Read the model definition and answer for the solid it produces. Units are mm, in the model's axes. Face numbers are marked on the shaded views. A direction names the side the tool comes from. Give positions to 0.01 mm unless a question says otherwise; leave off trailing zeros. Order: outer loops, then holes, each group sorted by start corner. A loop starts at its lowest first (then second) coordinate and runs counter-clockwise, first axis right, second up. Notation, with made-up numbers: (55, 56) -> (100, 56) arc R24 ccw to (100, 95) -> close; hole circle Ø2 at (-12.75, -24.75). An arc over 180 degrees is marked (long way). One line per item, written item: value. Start each with the question number.
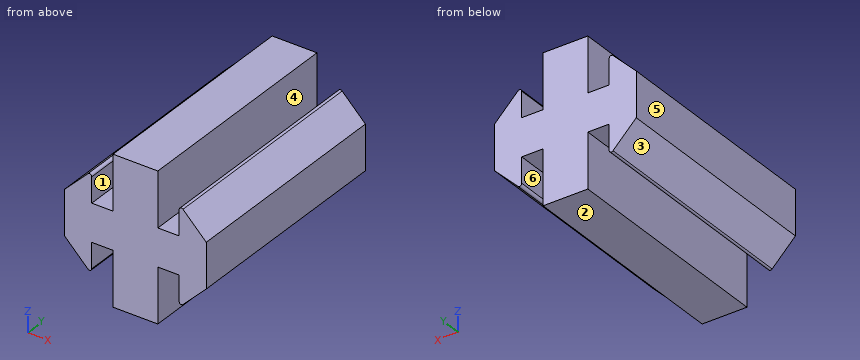
Autodesk Inventor part; units mm, degrees
ref_plane "YZ Plane" through (0, 0, 0) normal (1, 0, 0) x (0, 1, 0)
ref_plane "XZ Plane" through (0, 0, 0) normal (0, 1, 0) x (-1, 0, 0)
ref_plane "XY Plane" through (0, 0, 0) normal (0, 0, 1) x (1, 0, 0)
sketch "Sketch1" plane through (0, 0, 0) normal (0, 1, 0) x (-1, 0, 0)
  line L0 (0, 0) -> (5.08, 0)
  line L1 (5.08, 0) -> (5.08, -16.637)
  line L2 (5.08, -16.637) -> (0, -16.637)
  line L3 (0, -16.637) -> (0, 0)
  line L4 (0, -6.1892) -> (7.493, -6.1892)
  line L5 (7.493, -6.1892) -> (7.493, -10.4478)
  line L6 (7.493, -10.4478) -> (0, -10.4478)
  line L7 (10.5664, -5.7785) -> (10.5664, -10.8585)
  line L8 (7.493, -13.9319) -> (7.493, -2.7051)
  line L9 (7.493, -13.9319) -> (10.5664, -10.8585)
  line L10 (7.493, -2.7051) -> (10.5664, -5.7785)
  line L11 (0, -6.1892) -> (-2.413, -6.1892)
  line L12 (-2.413, -10.4478) -> (0, -10.4478)
  line L13 (-5.4864, -5.7785) -> (-5.4864, -10.8585)
  line L14 (-2.413, -13.9319) -> (-2.413, -2.7051)
  line L15 (-2.413, -13.9319) -> (-5.4864, -10.8585)
  line L16 (-2.413, -2.7051) -> (-5.4864, -5.7785)
  point P0 (-4.9276, -6.1892)
  dimension "d0" = 5.08
  dimension "d1" = 16.637
  dimension "d2" = 2.413
  dimension "d9" = 3.0734
  dimension "d12" = 0
  dimension "d16" = 11.2268
  dimension "d20" = 135
  dimension "d21" = 135
  dimension "d24" = 6.1893
  dimension "d25" = 16.637
  dimension "d26" = 3.4842
  dimension "d33" = 3.4842
  dimension "d34" = 3.0734
  dimension "d35" = 2.413
  dimension "d36" = 6.1893
  dimension "d37" = 5.08
  dimension "d38" = 5.08
  dimension "d39" = 135
  dimension "d40" = 135
extrude "Extrusion2" add sketch "Sketch1" along normal blind 25.4
fillet "Fillet1" radius 0.254 4 edges at (2.413, 12.7, -13.9319) (-7.493, 12.7, -13.9319) (2.413, 12.7, -2.7051) (-7.493, 12.7, -2.7051)
equation "\"d16\" = d15"
equation "\"d21\" = d20"
equation "\"d24\" = -0.5 * d4 + 0.5 * d25"
properties part number "20X20 lift conecter" material "PC/ABS Plastic"
Item 1: For a pull along X with two mould halves and no side action, classify the marked faces 1, 2 and 3 as +X half, -X half, draft (parallel to the pull), parting line (faces both ways), or undercut.
Item 2: Find section D-D on z = -14. Write down the section's boundary in (x, y), then the cut area to 3 significant figures.
Item 3: Find section C-C on x = -5.5. Write down the section's boundary in (y, z), then the cut area to 3 significant figures.
Item 4: Find the intervals of material crossed by line 1 (X direction, y = 10, z = -6); line 2 (X direction, y = 23.5, z = -5); line 3 (X direction, y = 20.75, z = -3), in increasing order. Write a range as from..to.
Item 5: Find section A-A on z = -5.5. Write down the section's boundary in (x, y), then the cut area to 3 significant figures.
Item 6: Find section B-B on y = 4.5. Write down the section's boundary in (x, z).
Item 7: A tool of negligible diameter and unlimited length cuts with its end or side. For the marked faces 4, 5 and 6, from which of +Z, -Z, +X, -X, +Y, -Y can it reach the whole face along a straight path? Write none if from no direction.
Item 8: Flat-ended cylindrical pins translate along their axes: pin 1 (1.5 mm diameter, centred on x = -4.5, y = 15, fed in from +Z); pin 2 (0.7 mm diameter, centred on x = 1, y = 11.5, fed in from -Z); pin 3 (1 mm diameter, centred on x = 2.5, y = 20, fed in from +Z); pin 4 (0.9 mm diameter, centred on y = 10.5, z = -4.5, fed in from +X). Find the tip coordinate at first contact, or state that the pin passes through.
Checks:
1. face 1: undercut
1. face 2: draft
1. face 3: -X half
2. outline: (-5.08, 0) -> (0, 0) -> (0, 25.4) -> (-5.08, 25.4) -> close
2. area: 129 mm2
3. outline: (0, -10.45) -> (25.4, -10.45) -> (25.4, -6.19) -> (0, -6.19) -> close
3. area: 108 mm2
4. line 1: -10.57..-7.49, -5.08..0, 2.41..5.49
4. line 2: -9.79..-7.49, -5.08..0, 2.41..4.71
4. line 3: -5.08..0
5. outline: (-10.29, 0) -> (-7.49, 0) -> (-7.49, 25.4) -> (-10.29, 25.4) -> close; (-5.08, 0) -> (0, 0) -> (0, 25.4) -> (-5.08, 25.4) -> close; (2.41, 0) -> (5.21, 0) -> (5.21, 25.4) -> (2.41, 25.4) -> close
5. area: 271 mm2
6. outline: (-10.57, -10.86) -> (-7.93, -13.5) arc R0.25 ccw to (-7.49, -13.32) -> (-7.49, -10.45) -> (-5.08, -10.45) -> (-5.08, -16.64) -> (0, -16.64) -> (0, -10.45) -> (2.41, -10.45) -> (2.41, -13.32) arc R0.25 ccw to (2.85, -13.5) -> (5.49, -10.86) -> (5.49, -5.78) -> (2.85, -3.14) arc R0.25 ccw to (2.41, -3.32) -> (2.41, -6.19) -> (0, -6.19) -> (0, 0) -> (-5.08, 0) -> (-5.08, -6.19) -> (-7.49, -6.19) -> (-7.49, -3.32) arc R0.25 ccw to (-7.93, -3.14) -> (-10.57, -5.78) -> close
7. face 4: +Z, +Y, -Y
7. face 5: +Z, -Z, -X, +Y, -Y
7. face 6: -Z, +Y, -Y
8. pin 1: z = 0
8. pin 2: z = -10.45
8. pin 3: z = -3.06
8. pin 4: x = 4.66
